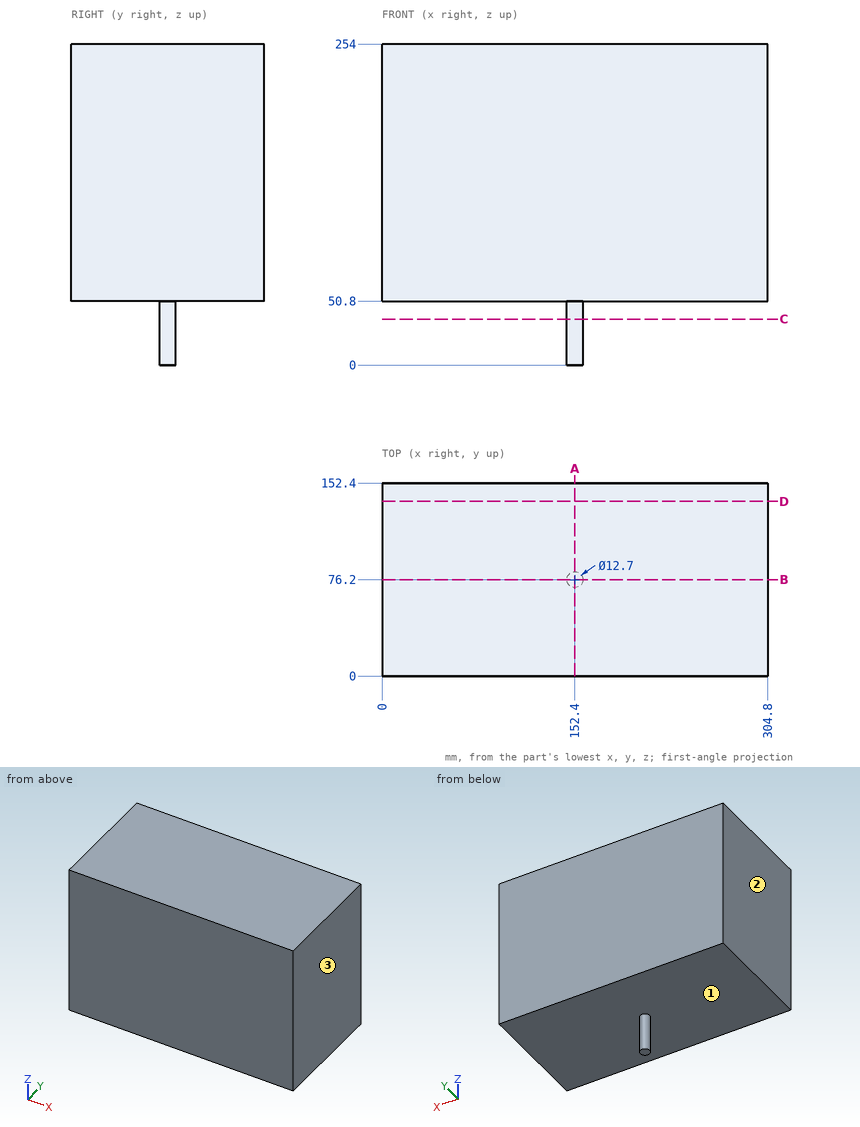
Could you check a few things on this drawing? It's one solid part, dimensions in mm from its lowest x, y, z. Coordinates: 2 decimals unless noted, no trailing zeros. Order: outer loops, then holes, each group sorted by start corner. A loop starts at its lowest first (then second) coordinate and runs counter-clockwise, first axis right, second up. Notation, with made-up numbers: (2, 38.5) - (53, 38.5) arc R11 cw to (53, 55.5) - close; hole circle Ø8 at (-23, 62.5). An arc over 180 degrees is marked (long way). One line per question, with ' | ' between items. Start each with the question number.
1. Please list where these lines run through material, in increasing order: line 1 along Z through (x, y) = (83.5, 114); line 2 along X through (y, z) = (78.5, 42). Write a range as [from, to].
2. If we section it at A-A (x = 152.4): Write out the boundary of the cut face in (y, z), and give its area (3 significant figures).
3. If we section it at B-B (y = 76.2): Write out the boundary of the cut face in (x, z), and give its area (3 significant figures).
4. If we mould it in two halves opening along X, with no side actions, what happens to the marked faces 1, 2 and 3? For each: released by +X, released by -X, zero draft, split by the parting line, or undercut.
5. If we section it at D-D (y = 138): Write out the boundary of the cut face in (x, z).
6. If we section it at C-C (z = 36.5): Write out the boundary of the cut face in (x, y).
Model answer:
1) line 1: z = [50.8, 254] | line 2: x = [146.48, 158.32]
2) outline: (0, 50.8) - (69.85, 50.8) - (69.85, 0) - (82.55, 0) - (82.55, 50.8) - (152.4, 50.8) - (152.4, 254) - (0, 254) - close | area: 31,600 mm²
3) outline: (0, 50.8) - (146.05, 50.8) - (146.05, 0) - (158.75, 0) - (158.75, 50.8) - (304.8, 50.8) - (304.8, 254) - (0, 254) - close | area: 62,600 mm²
4) face 1: zero draft | face 2: released by -X | face 3: released by +X
5) outline: (0, 50.8) - (304.8, 50.8) - (304.8, 254) - (0, 254) - close
6) outline: circle Ø12.7 at (152.4, 76.2)
